Source: CAD feature listing. Evaluate the final solid. Frame: model axes, mm. Face numbers are marked on the shaded views. A direction names the side the tool comes from. Coordinates: 2 decimals unless noted, no trailing zeros. Write each loop counter-clockwise with the first axis right and the second up, starting at its lowest first coordinate (ties: lowest second). Pieces come first, ordered by that corner, then holes. Notation, with made-up numbers: M -9.5,59 L 45.5,59 A23 cw 45.5,71 Z; hole C 39.5,86 d5. An arc over 180 degrees is marked long. One line per item, written item: value. Start each with the question number.
Item 1: Cut plane C-C, the plane x = -3.25. Output: boundary loops of the cut face in (y, z), then the cut area to 3 significant figures.
Item 2: Cut plane A-A, the plane y = 1.5. Output: boundary loops of the cut face in (x, z).
Item 3: Cut plane D-D, the plane y = 3.7. Output: boundary loops of the cut face in (x, z), then the cut area to 3 significant figures.
Item 4: Mould query, pull axis X, two halves, no side actions, for the marked faces 1, 2 and 3. Classes: released by +X, released by -X, zero draft, split by the parting line, or undercut.
Item 5: Set-up query: the marked faces 4, 5 and 6. Return all of +Z, -Z, +X, -X, +Y, -Y with unobstructed straight access to the full face (end or side cutting, diameter ignored); none if empty.
Item 6: Pin query (flat end, axial travel): P1, Ø1.6, axis at y = 5, z = -12, coming from the -X side; P2, Ø0.8, axis at x = -8, y = 4, coming from the -Z side; P3, Ø5.5, axis at x = -5.5, z = -2, coming from the +Y side; P4, Ø0.9, axis at x = -18, z = -12, coming from the -Y side. Return the tip coordinate at first contact, or that it passes through.
Item 7: Cut plane B-B, the plane z = -12.5. Output: boundary loops of the cut face in (x, y) (3 decimals), then the cut area to 3 significant figures.
Item 8: Ray query, L1, parallel to X at y = 3.55, z = -0.75; L2, parallel to Z at x = -6.75, y = 2.45; L3, parallel to Z at x = -12.5, y = 4.25. Return the intervals inside material, ascending. Write a range as from..to.
```python
from build123d import *

# Parameters (mm, degrees)
SKETCH2_W           = 15.9999934
SKETCH2_H           = 15
BOSS_EXTRUDE2_DEPTH = 6
SKETCH6_W           = 16
SKETCH6_H           = 7
CUT_EXTRUDE3_DEPTH  = 2
SKETCH7_W           = 6
SKETCH7_H           = 3
CUT_EXTRUDE4_DEPTH  = 23.293492073
SKETCH12_R          = 0.635
CUT_EXTRUDE5_DEPTH  = 100
SKETCH13_W          = 8
SKETCH13_H          = 2
BOSS_EXTRUDE3_DEPTH = 3


with BuildPart() as part:
    # Sketch2 → Boss-Extrude2 (new body)
    with BuildSketch(Plane(origin=(0, 0, 0), x_dir=(1, 0, 0), z_dir=(0, 1, 0))):
        with Locations((-7.9999967, 7.5)):
            Rectangle(SKETCH2_W, SKETCH2_H)
    extrude(amount=BOSS_EXTRUDE2_DEPTH)

    # Sketch6 → Cut-Extrude3 (cut)
    with BuildSketch(Plane(origin=(0, 6, 0), x_dir=(1, 0, 0), z_dir=(0, 1, 0))):
        with Locations((-7.9999934, 3.5)):
            Rectangle(SKETCH6_W, SKETCH6_H)
    extrude(amount=-CUT_EXTRUDE3_DEPTH, mode=Mode.SUBTRACT)

    # Sketch7 → Cut-Extrude4 (cut, through all)
    with BuildSketch(Plane(origin=(0, 4, 0), x_dir=(1, 0, 0), z_dir=(0, 1, 0))):
        with Locations((-8, 1.5)):
            Rectangle(SKETCH7_W, SKETCH7_H)
    extrude(amount=-CUT_EXTRUDE4_DEPTH, mode=Mode.SUBTRACT)

    # Sketch12 → Cut-Extrude5 (cut)
    with BuildSketch(Plane(origin=(0, 0, -15), x_dir=(-1, 0, 0), z_dir=(0, 0, -1))):
        with Locations((7.9999967, 4)):
            Circle(SKETCH12_R)
    extrude(amount=-CUT_EXTRUDE5_DEPTH, mode=Mode.SUBTRACT)

    # Sketch13 → Boss-Extrude3 (add)
    with BuildSketch(Plane.ZY.offset(15.9999934)):
        with Locations((-11, 3)):
            Rectangle(SKETCH13_W, SKETCH13_H)
    extrude(amount=BOSS_EXTRUDE3_DEPTH)


solid = part.part
```
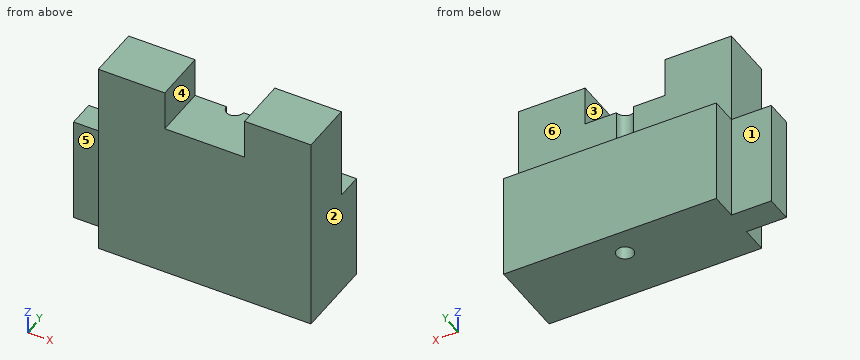
From the geometry:
1. outline: M 0,-15 L 6,-15 L 6,-7 L 4,-7 L 4,0 L 0,0 Z
1. area: 76.0 mm²
2. outline: M -16,-15 L 0,-15 L 0,0 L -5,0 L -5,-3 L -11,-3 L -11,0 L -16,0 Z
3. outline: M -19,-15 L -8.56,-15 L -8.56,-3 L -11,-3 L -11,0 L -16,0 L -16,-7 L -19,-7 Z; M -7.44,-15 L 0,-15 L 0,0 L -5,0 L -5,-3 L -7.44,-3 Z
3. area: 233 mm²
4. face 1: zero draft
4. face 2: released by +X
4. face 3: undercut
5. face 4: +Z, +Y, -Y
5. face 5: +Z, -Z, -X, -Y
5. face 6: +Z, +X, -X, +Y
6. P1: stops at x = -16
6. P2: passes through
6. P3: stops at y = 4
6. P4: stops at y = 2
7. outline: M -19,2 L -16,2 L -16,0 L 0,0 L 0,6 L -16,6 L -16,4 L -19,4 Z; hole C -8,4 d1.27
7. area: 101 mm²
8. L1: x = -16..-11, -5..0
8. L2: z = -15..-3
8. L3: z = -15..-7
